```python
from build123d import *

# Parameters (mm, degrees)
SKETCH8_R           = 100
BOSS_EXTRUDE4_DEPTH = 40
CUT_EXTRUDE1_DEPTH  = 147.969384567


with BuildPart() as part:
    # Sketch8 → Boss-Extrude4 (new body)
    with BuildSketch(Plane(origin=(0, 0, 0), x_dir=(1, 0, 0), z_dir=(0, 1, 0))):
        with Locations(Location((0, 0, 0), (0, 0, 270))):
            Circle(SKETCH8_R)
    extrude(amount=BOSS_EXTRUDE4_DEPTH)

    # Sketch6 → Cut-Extrude1 (cut, through all)
    with BuildSketch(Plane(origin=(0, 0, 0), x_dir=(1, 0, 0), z_dir=(0, 1, 0))):
        Polygon((-0.9689411, -22.736267788), (0.9689411, -22.736267788), (2.2189411, -24.901331298), (4.303288018, -24.645405677), (4.950335631, -22.230591111), (6.822186096, -21.72903029), (8.589953049, -23.496797243), (10.537039143, -22.710123397), (10.537039143, -20.210123397), (12.215294358, -19.241182297), (14.380357867, -20.491182297), (16.057492438, -19.227370749), (15.410444825, -16.812556183), (16.78073447, -15.442266539), (19.195549035, -16.089314151), (20.488438134, -14.434491569), (19.238438134, -12.269428059), (20.207379233, -10.591172845), (22.707379233, -10.591172845), (23.527914603, -8.658112653), (21.76014765, -6.8903457), (22.261708471, -5.018495235), (24.676523036, -4.371447622), (24.968786548, -2.291884678), (22.803723039, -1.041884678), (22.803723039, 0.895997521), (24.968786548, 2.145997521), (24.712860927, 4.23034444), (22.298046362, 4.877392053), (21.796485541, 6.749242517), (23.564252494, 8.51700947), (22.777578648, 10.464095565), (20.277578648, 10.464095565), (19.308637548, 12.142350779), (20.558637548, 14.307414289), (19.294826, 15.98454886), (16.880011434, 15.337501247), (15.509721789, 16.707790891), (16.156769402, 19.122605457), (14.50194682, 20.415494555), (12.33688331, 19.165494555), (10.658628096, 20.134435655), (10.658628096, 22.634435655), (8.725567904, 23.454971025), (6.957800951, 21.687204072), (5.085950486, 22.188764892), (4.438902873, 24.603579458), (2.359339929, 24.89584297), (1.109339929, 22.730779461), (-0.828542271, 22.730779461), (-2.078542271, 24.89584297), (-4.162889189, 24.639917349), (-4.809936802, 22.225102783), (-6.681787267, 21.723541963), (-8.44955422, 23.491308916), (-10.396640314, 22.70463507), (-10.396640314, 20.20463507), (-12.074895529, 19.23569397), (-14.239959038, 20.48569397), (-15.917093609, 19.221882421), (-15.270045996, 16.807067856), (-16.640335641, 15.436778211), (-19.055150206, 16.083825824), (-20.348039305, 14.429003241), (-19.098039305, 12.263939732), (-20.066980404, 10.585684518), (-22.566980404, 10.585684518), (-23.387515774, 8.652624325), (-21.619748821, 6.884857372), (-22.121309642, 5.013006908), (-24.536124207, 4.365959295), (-24.828387719, 2.28639635), (-22.66332421, 1.03639635), (-22.66332421, -0.901485849), (-24.828387719, -2.151485849), (-24.572462098, -4.235832767), (-22.157647532, -4.88288038), (-21.656086712, -6.754730845), (-23.423853665, -8.522497798), (-22.637179819, -10.469583893), (-20.137179819, -10.469583893), (-19.168238719, -12.147839107), (-20.418238719, -14.312902616), (-19.154427171, -15.990037187), (-16.739612605, -15.342989575), (-15.36932296, -16.713279219), (-16.016370573, -19.128093785), (-14.361547991, -20.420982883), (-12.196484481, -19.170982883), (-10.518229267, -20.139923983), (-10.518229267, -22.639923983), (-8.585169075, -23.460459352), (-6.817402122, -21.6926924), (-4.945551657, -22.19425322), (-4.298504044, -24.609067786), (-2.2189411, -24.901331298), align=None)
    extrude(amount=CUT_EXTRUDE1_DEPTH, mode=Mode.SUBTRACT)


solid = part.part
```
Work out the finished part from the listing and answer in its coordinate system (mm). Coordinates: 2 decimals unless noted, no trailing zeros. Loops run counter-clockwise (first coordinate to the right, second up) from the corner with the lowest first, then second, coordinate; pieces in that order, holes last. Notation, with made-up numbers: (27.5, -31.5) - (78.5, -31.5) arc R28 ccw to (78.5, -6.5) - close; hole circle Ø6 at (-1.75, 33). An arc over 180 degrees is marked (long way). Use a Markdown table: item, result.
Item 1: Given pin 1 Ø1.5 at (y, z) = (25, -67) entering from +X; pin 2 Ø12 at (y, z) = (6.5, 32.5) entering from +X; pin 3 Ø0.8 at (x, y) = (-21.5, 27) entering from +Z, each flat-ended and moving along its own axis, determine where each tip first touches the part or whether it passes through.
Evaluation:
| item | result |
|---|---|
| pin 1 | stops at x = 74.91 |
| pin 2 | stops at x = 96.42 |
| pin 3 | stops at z = 97.75 |
Item 2: Consider probe 1 along Z at (x, y) = (-24, 10); probe 2 along Z at (x, y) = (-14, 17); probe 3 along X at (y, z) = (24, -6). Determine where each line is inside the solid, lowest interval first. Write a range as from..to.
Evaluation:
| item | result |
|---|---|
| probe 1 | z = -97.08..-4.51, -1.81..1.67, 4.39..97.08 |
| probe 2 | z = -99.02..-20.35, 20.21..99.02 |
| probe 3 | x = -99.82..-21.86, 22..99.82 |
Item 3: Find section A-A, the plane x = 62.5. Determine the outline of the cut face in (y, z).
Evaluation:
| item | result |
|---|---|
| outline | (0, -78.06) - (40, -78.06) - (40, 78.06) - (0, 78.06) - close |
Item 4: Find section B-B, the plane z = -75.5. Determine the outline of the cut face in (x, y).
Evaluation:
| item | result |
|---|---|
| outline | (-65.57, 0) - (65.57, 0) - (65.57, 40) - (-65.57, 40) - close |
